Model file for the job. Use its own axes, mm. Face numbers are marked on the shaded views. A direction names the side the tool comes from. Give positions to 0.01 mm unless a question says otherwise; leave off trailing zeros. Write each loop counter-clockwise with the first axis right and the second up, starting at its lowest first coordinate (ties: lowest second). Pieces come first, ordered by that corner, then holes. Notation, with made-up numbers: M 53,89.5 L 96,89.5 A12 ccw 96,94.5 Z; hole C 67,-39 d7. An arc over 180 degrees is marked long. Answer as a JSON object with one key per item and string values. Group by question number.
```python
from build123d import *

# Parameters (mm, degrees)
F1_DEPTH = 127
F3_DEPTH = 101.6


with BuildPart() as f1:
    # F0 (on Top) → F1 (new body)
    with BuildSketch(Plane.XY):
        with BuildLine():
            Line((96.324614, 76.2), (-106.875386, 76.2))
            Line((-106.875386, 76.2), (-106.875386, -76.2))
            Line((-106.875386, -76.2), (96.324614, -76.2))
            Line((96.324614, -76.2), (96.324614, -50.8))
            ThreePointArc((96.324614, -50.8), (45.524614, 0), (96.324614, 50.8))
            Line((96.324614, 50.8), (96.324614, 76.2))
        make_face()
    extrude(amount=F1_DEPTH)

    # F2 (on face) → F3 (cut)
    with BuildSketch(Plane(origin=(-106.875386, 0, 0), x_dir=(0, -1, 0), z_dir=(-1, 0, 0))):
        with BuildLine():
            Line((76.2, 127), (-25.4, 127))
            ThreePointArc((-25.4, 127), (10.129609, 60.929609), (76.2, 25.4))
            Line((76.2, 25.4), (76.2, 127))
        make_face()
    extrude(amount=-F3_DEPTH, mode=Mode.SUBTRACT)


solid = f1.part
```
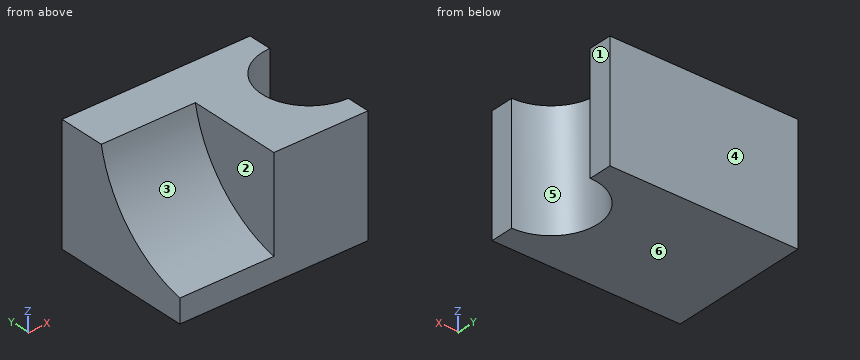
Q1. 3-axis set-ups, long thin cutter, end or side, ignore diameter. For the marked faces 1 and 2: which of +Z, -Z, +X, -X, +Y, -Y reach the whole face in a straight line?
Q2. Two-plate mould, pull along Y, no slides. Class the marked faces 3, 4, 5 and 6: +Y half, -Y half, draft (parallel to the pull), parting line (faces both ways), or undercut.
Q3. Slice it at B-B, the plane x = -71. Write the cut outline in (y, z).
Q4. Wall check: L1, parallel to Y at x = 50, z = 24.5; L2, parallel to Y at x = 66.5, z = 17.5; L3, parallel to X at y = -60.5, z = 114. Give the ranges that are in metal, low to high.
Q5. Slice it at D-D, the plane z = 59. Write the cut outline in (x, y), then the cut area to 3 significant figures.
Q6. Slice it at C-C, the plane y = 0. Write the cut outline in (x, z), then the cut area to 3 significant figures.
Q7. Drop flat-ended pins along their axis: P1, Ø2, axis at y = -20, z = 56, coming from the +X side; P2, Ø4, axis at x = -52.5, z = 35, coming from the -Y side; P3, Ø1, axis at y = -59.5, z = 65.5, coming from the -X side. Give the stop position or say it passes through.
Q8. Slice it at A-A, the plane z = 118. Write the cut outline in (x, y).
Solved:
{
 "1": {"face 1": "+Z, -Z, +X, +Y, -Y", "face 2": "+Z, -X, -Y"},
 "2": {"face 3": "-Y half", "face 4": "+Y half", "face 5": "undercut", "face 6": "draft"},
 "3": {"outline": "M -76.2,0 L 76.2,0 L 76.2,127 L 25.4,127 A130.3 cw -76.2,25.4 Z"},
 "4": {"L1": "y = -76.2 to -20.85, 20.85 to 76.2", "L2": "y = -76.2 to -41.12, 41.12 to 76.2", "L3": "x = -5.28 to 96.32"},
 "5": {"outline": "M -106.88,-12.1 L -5.28,-12.1 L -5.28,-76.2 L 96.32,-76.2 L 96.32,-50.8 A50.8 cw 96.32,50.8 L 96.32,76.2 L -106.88,76.2 Z", "area": "20,400 mm²"},
 "6": {"outline": "M -106.88,0 L 45.52,0 L 45.52,127 L -5.28,127 L -5.28,72.32 L -106.88,72.32 Z", "area": "13,800 mm²"},
 "7": {"P1": "stops at x = 50.07", "P2": "stops at y = -51.65", "P3": "stops at x = -5.28"},
 "8": {"outline": "M -106.88,23.23 L -5.28,23.23 L -5.28,-76.2 L 96.32,-76.2 L 96.32,-50.8 A50.8 cw 96.32,50.8 L 96.32,76.2 L -106.88,76.2 Z"}
}
